Part model, mm, in its own coordinate system. Face numbers are marked on the shaded views. A direction names the side the tool comes from. Round coordinates to 2 decimals unless told otherwise and drop trailing zeros. Write each loop counter-clockwise with the first axis right and the second up, starting at its lowest first coordinate (ties: lowest second). Pieces come first, ordered by that corner, then holes.
1) Saw through at D-D on y = 0. Write the cut outline in (x, z).
2) Flat gauge pins, fed straight in: pin 1 (0.5 mm diameter, centred on y = -109.5, z = 67.5, fed in from -X); pin 2 (12 mm diameter, centred on y = 68.5, z = 78.5, fed in from -X); pin 3 (17.5 mm diameter, centred on x = 118, y = 21.5, fed in from +Z). Where does each tip first touch, or does it go through?
3) Saw through at B-B on z = 300.5. Write the cut outline in (x, y), and give its area (3 significant figures).
4) Drill centre lines: L1, parallel to Y at x = -22.5, z = 50.5; L2, parallel to Y at x = -37.5, z = 189; L3, parallel to X at y = 17, z = 277. Where is each one in solid material? Low to high.
5) Saw through at A-A on x = 0. Write the cut outline in (y, z), and give its area (3 significant figures).
6) Saw through at C-C on y = -50. Write the cut outline in (x, z).
7) Which spindle directions (+Z, -Z, +X, -X, +Y, -Y) get a long thin tool onto all of the face, cutting with end or side? Do the marked faces 1, 2 and 3. Say none if no direction does.
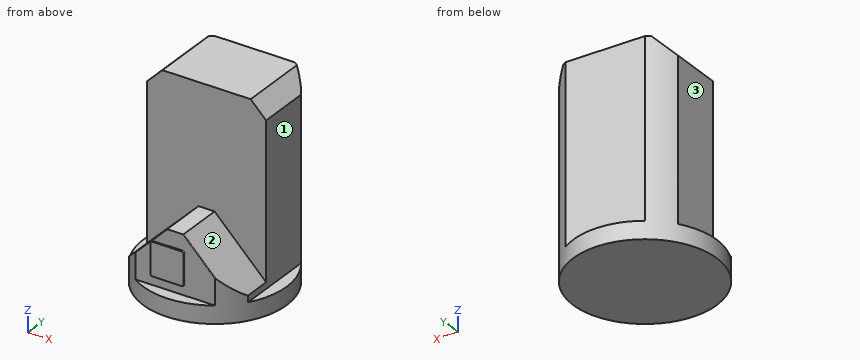
```python
from build123d import *

# Parameters (mm, degrees)
SKETCH3_R             = 130
BOSS_EXTRUDE1_DEPTH   = 352
CUT_EXTRUDE2_DEPTH    = 320
CUT_EXTRUDE3_DEPTH    = 320
CUT_EXTRUDE4_DEPTH    = 85
CUT_EXTRUDE5_DEPTH    = 85
CUT_EXTRUDE7_REACH    = 354
CUT_EXTRUDE8_REACH    = 354
CUT_EXTRUDE9_DEPTH    = 285
SKETCH22_W            = 60
SKETCH22_H            = 60
BOSS_EXTRUDE3_DEPTH   = 2
FILLET1_R             = 3
FILLET2_R             = 3
FILLET4_R             = 1
FILLET5_R             = 1
BODY_MOVE_COPY2_ANGLE = 90
BODY_MOVE_COPY3_ANGLE = 90
BODY_MOVE_COPY4_ANGLE = 180


with BuildPart() as part:
    # Sketch3 → Boss-Extrude1 (new body)
    with BuildSketch(Plane(origin=(0, 0, 0), x_dir=(1, 0, 0), z_dir=(0, 1, 0))):
        Circle(SKETCH3_R)
    extrude(amount=BOSS_EXTRUDE1_DEPTH)

    # Sketch11 → Cut-Extrude2 (cut)
    with BuildSketch(Plane(origin=(0, 352, 0), x_dir=(1, 0, 0), z_dir=(0, 1, 0))):
        with BuildLine():
            Line((72.360210061, -108), (0, -108))
            Line((0, -108), (-72.360210061, -108))
            ThreePointArc((-72.360210061, -108), (0, -130), (72.360210061, -108))
        make_face()
        with BuildLine():
            Line((-72.360210061, 108), (72.360210061, 108))
            ThreePointArc((72.360210061, 108), (0, 130), (-72.360210061, 108))
        make_face()
    extrude(amount=-CUT_EXTRUDE2_DEPTH, mode=Mode.SUBTRACT)

    # Sketch11<4> → Cut-Extrude3 (cut)
    with BuildSketch(Plane(origin=(0, 352, 0), x_dir=(1, 0, 0), z_dir=(0, 1, 0))):
        with BuildLine():
            ThreePointArc((-108, 72.360210061), (-130, 0), (-108, -72.360210061))
            Line((-108, -72.360210061), (-108, 72.360210061))
        make_face()
        with BuildLine():
            Line((108, 72.360210061), (108, 0))
            Line((108, 0), (108, -72.360210061))
            ThreePointArc((108, -72.360210061), (124.378454726, -37.815340802), (130, 0))
            ThreePointArc((130, 0), (124.378454726, 37.815340802), (108, 72.360210061))
        make_face()
    extrude(amount=-CUT_EXTRUDE3_DEPTH, mode=Mode.SUBTRACT)

    # Sketch12 → Cut-Extrude4 (cut)
    with BuildSketch(Plane.ZY.offset(108)):
        Polygon((-72.360210061, 137), (0, 137), (72.360210061, 137), (72.360210061, 352), (-72.360210061, 352), align=None)
    extrude(amount=-CUT_EXTRUDE4_DEPTH, mode=Mode.SUBTRACT)

    # Sketch14 → Cut-Extrude5 (cut)
    with BuildSketch(Plane.ZY.offset(108)):
        Polygon((-72.360210061, 79.254886678), (-14.615096739, 137), (-72.360210061, 137), align=None)
        Polygon((72.360210061, 137), (14.615096739, 137), (72.360210061, 79.254886678), align=None)
    extrude(amount=-CUT_EXTRUDE5_DEPTH, mode=Mode.SUBTRACT)

    # Cut-Extrude7: up to this face of the body (flat: up to its plane)
    cut_extrude7_end = Plane(part.part.faces().sort_by_distance((-65.5, 108.127443339, -43.4876534))[0])
    # Sketch15 → Cut-Extrude7 (cut, up to the picked face)
    with BuildSketch(Plane(origin=(0, 352, 0), x_dir=(1, 0, 0), z_dir=(0, 1, 0)), mode=Mode.PRIVATE) as cut_extrude7_sk1:
        with BuildLine():
            Line((-108, 72.360210061), (-23, 72.360210061))
            Line((-23, 72.360210061), (-23, 108))
            Line((-23, 108), (-72.360210061, 108))
            ThreePointArc((-72.360210061, 108), (-91.923881554, 91.923881554), (-108, 72.360210061))
        make_face()
    cut_extrude7_tool1 = split(extrude(cut_extrude7_sk1.sketch, amount=-CUT_EXTRUDE7_REACH, mode=Mode.PRIVATE), bisect_by=cut_extrude7_end, keep=Keep.BOTH, mode=Mode.PRIVATE)
    add(cut_extrude7_tool1.solids().sort_by_distance((-58.500557, 352, -88.680695))[0], mode=Mode.SUBTRACT)

    # Cut-Extrude8: up to this face of the body (flat: up to its plane)
    cut_extrude8_end = Plane(part.part.faces().sort_by_distance((-65.5, 108.127443339, 43.4876534))[0])
    # Sketch15<4> → Cut-Extrude8 (cut, up to the picked face)
    with BuildSketch(Plane(origin=(0, 352, 0), x_dir=(1, 0, 0), z_dir=(0, 1, 0)), mode=Mode.PRIVATE) as cut_extrude8_sk1:
        with BuildLine():
            Line((-23, -108), (-23, -72.360210061))
            Line((-23, -72.360210061), (-108, -72.360210061))
            ThreePointArc((-108, -72.360210061), (-91.923881554, -91.923881554), (-72.360210061, -108))
            Line((-72.360210061, -108), (-23, -108))
        make_face()
    cut_extrude8_tool1 = split(extrude(cut_extrude8_sk1.sketch, amount=-CUT_EXTRUDE8_REACH, mode=Mode.PRIVATE), bisect_by=cut_extrude8_end, keep=Keep.BOTH, mode=Mode.PRIVATE)
    add(cut_extrude8_tool1.solids().sort_by_distance((-58.500557, 352, 88.680695))[0], mode=Mode.SUBTRACT)

    # Sketch18 → Cut-Extrude9 (cut)
    with BuildSketch(Plane.ZY.offset(23)):
        Polygon((-108, 324), (-80, 352), (-108, 352), align=None)
        Polygon((108, 352), (80, 352), (108, 324), align=None)
    extrude(amount=-CUT_EXTRUDE9_DEPTH, mode=Mode.SUBTRACT)

    # Sketch22 → Boss-Extrude3 (add)
    with BuildSketch(Plane.ZY.offset(108)):
        with Locations((-13.4876534, 78.127443339)):
            Rectangle(SKETCH22_W, SKETCH22_H)
    extrude(amount=BOSS_EXTRUDE3_DEPTH)

    # Fillet1
    fillet1_edges = [part.edges().sort_by_distance(p)[0] for p in [
        (-109, 108.127443339, -43.4876534),
    ]]
    fillet(fillet1_edges, radius=FILLET1_R)

    # Fillet2
    fillet2_edges = [part.edges().sort_by_distance(p)[0] for p in [
        (-109, 48.127443339, 16.5123466),
        (-109, 108.127443339, 16.5123466),
        (-109, 48.127443339, -43.4876534),
    ]]
    fillet(fillet2_edges, radius=FILLET2_R)

    # Fillet4
    fillet4_edges = [part.edges().sort_by_distance(p)[0] for p in [
        (-108, 122.56372167, -29.051375069),
        (-108, 93.691165009, -57.92393173),
        (-108, 108.127443339, 43.4876534),
    ]]
    fillet(fillet4_edges, radius=FILLET4_R)

    # Fillet5
    fillet5_edges = [part.edges().sort_by_distance(p)[0] for p in [
        (-108, 78.127443339, -43.4876534),
        (-108, 108.127443339, -13.4876534),
        (-108, 107.248763683, -42.608973743),
        (-108, 48.127443339, -13.4876534),
        (-108, 78.127443339, 16.5123466),
        (-108, 49.006122995, -42.608973743),
        (-108, 49.006122995, 15.633666944),
        (-108, 107.248763683, 15.633666944),
    ]]
    fillet(fillet5_edges, radius=FILLET5_R)


with BuildPart() as part_1:
    # Body-Move/Copy2: moved
    add(part.part.rotate(Axis((0, 0, 0), (1, 0, 0)), BODY_MOVE_COPY2_ANGLE))


with BuildPart() as part_2:
    # Body-Move/Copy3: moved
    add(part_1.part.rotate(Axis((0, 0, 0), (0, 0, -1)), BODY_MOVE_COPY3_ANGLE))


with BuildPart() as part_3:
    # Body-Move/Copy4: moved
    add(part_2.part.rotate(Axis((0, 0, 0), (0, 0, 1)), BODY_MOVE_COPY4_ANGLE))


solid = part_3.part
```
Completed:
1. outline: (-130, 0) - (130, 0) - (130, 32) - (108, 32) - (108, 324) - (80, 352) - (-80, 352) - (-108, 324) - (-108, 32) - (-130, 32) - close
2. pin 1: stops at x = -43.49
2. pin 2: stops at x = -108
2. pin 3: stops at z = 32
3. outline: (-108, -23) - (108, -23) - (108, 72.36) arc R130 ccw to (72.36, 108) - (-72.36, 108) arc R130 ccw to (-108, 72.36) - close
3. area: 27,200 mm2
4. L1: y = -110 to 108
4. L2: y = -23 to 108
4. L3: x = -108 to 108
5. outline: (-130, 0) - (130, 0) - (130, 32) - (108, 32) - (108, 352) - (-23, 352) - (-23, 137) - (-108, 137) - (-108, 109.13) arc R1 cw to (-109, 108.13) - (-110, 108.13) - (-110, 48.13) - (-109, 48.13) arc R1 cw to (-108, 47.13) - (-108, 32) - (-130, 32) - close
5. area: 59,300 mm2
6. outline: (-120, 0) - (120, 0) - (120, 32) - (108, 32) - (108, 43.62) - (14.62, 137) - (-14.62, 137) - (-108, 43.62) - (-108, 32) - (-120, 32) - close
7. face 1: +Z, +X, +Y, -Y
7. face 2: +Z, +X, -Y
7. face 3: +Z, -X, +Y, -Y
